For this review, take the finished solid that the model builds, in its own axes (mm). A direction names the side the tool comes from. Round coordinates to 2 decimals unless told otherwise and drop trailing zeros. Write each loop counter-clockwise with the first axis right and the second up, starting at its lowest first coordinate (ties: lowest second). Pieces come first, ordered by that corner, then holes.
from build123d import *

# Parameters (mm, degrees)
ESQUISSE1_R             = 17.7
ESQUISSE1_R_2           = 12.7
BOSS_EXTRU_1_DEPTH      = 12.7
BOSS_EXTRU_2_DEPTH      = 12.7
ESQUISSE3_R             = 3.175
ENL_V_MAT_EXTRU_1_DEPTH = 62.63061651
ESQUISSE4_R             = 3.175
ENL_V_MAT_EXTRU_2_DEPTH = 62.63061651
ESQUISSE5_R             = 3.175
ENL_V_MAT_EXTRU_3_DEPTH = 49.65374434
CONG_1_R                = 1


with BuildPart() as part:
    # Esquisse1 → Boss.-Extru.1 (new body)
    with BuildSketch(Plane.XY):
        Circle(ESQUISSE1_R)
        Circle(ESQUISSE1_R_2, mode=Mode.SUBTRACT)
    extrude(amount=BOSS_EXTRU_1_DEPTH)

    # Esquisse2 → Boss.-Extru.2 (add)
    with BuildSketch(Plane.XY.offset(12.7)):
        Polygon((28.45374434, 23.760125373), (11.133236264, 13.760125373), (6.087254248, 16.620328989), (25.95374434, 28.090252392), align=None)
        Polygon((17.483236264, 2.761602745), (17.437254248, -3.038447676), (37.30374434, 8.431475726), (34.80374434, 12.761602745), align=None)
        Polygon((11.35, -36.521728118), (11.35, -13.581881313), (6.35, -16.521728118), (6.35, -36.521728118), align=None)
        Polygon((-6.35, -16.521728118), (-11.35, -13.581881313), (-11.35, -36.521728118), (-6.35, -36.521728118), align=None)
        Polygon((-37.30374434, 8.431475726), (-17.437254248, -3.038447676), (-17.483236264, 2.761602745), (-34.80374434, 12.761602745), align=None)
        Polygon((-11.133236264, 13.760125373), (-6.087254248, 16.620328989), (-25.95374434, 28.090252392), (-28.45374434, 23.760125373), align=None)
    extrude(amount=-BOSS_EXTRU_2_DEPTH)

    # Esquisse3 → Enlèv. mat.-Extru.1 (cut, through all)
    with BuildSketch(Plane(origin=(5.675, 9.829388333, 0), x_dir=(0.866025404, -0.5, 0), z_dir=(0.5, 0.866025404, 0))):
        with Locations((-28.584228118, -6.35)):
            Circle(ESQUISSE3_R)
    extrude(amount=-ENL_V_MAT_EXTRU_1_DEPTH, mode=Mode.SUBTRACT)

    # Esquisse4 → Enlèv. mat.-Extru.2 (cut, through all)
    with BuildSketch(Plane(origin=(-5.675, 9.829388333, 0), x_dir=(0.866025404, 0.5, 0), z_dir=(-0.5, 0.866025404, 0))):
        with Locations((28.584228118, -6.35)):
            Circle(ESQUISSE4_R)
    extrude(amount=-ENL_V_MAT_EXTRU_2_DEPTH, mode=Mode.SUBTRACT)

    # Esquisse5 → Enlèv. mat.-Extru.3 (cut, through all)
    with BuildSketch(Plane(origin=(11.35, 0, 0), x_dir=(0, 0, -1), z_dir=(1, 0, 0))):
        with Locations((-6.35, -28.584228118)):
            Circle(ESQUISSE5_R)
    extrude(amount=-ENL_V_MAT_EXTRU_3_DEPTH, mode=Mode.SUBTRACT)

    # Congé1
    cong_1_edges = [part.edges().sort_by_distance(p)[0] for p in [
        (25.95374434, 28.090252392, 6.35),
        (28.45374434, 23.760125373, 6.35),
        (11.133236264, 13.760125373, 6.35),
        (6.087254248, 16.620328989, 6.35),
        (17.483236264, 2.761602745, 6.35),
        (34.80374434, 12.761602745, 6.35),
        (37.30374434, 8.431475726, 6.35),
        (17.437254248, -3.038447676, 6.35),
        (11.35, -36.521728118, 6.35),
        (6.35, -36.521728118, 6.35),
        (6.35, -16.521728118, 6.35),
        (11.35, -13.581881313, 6.35),
        (-6.35, -16.521728118, 6.35),
        (-6.35, -36.521728118, 6.35),
        (-11.35, -36.521728118, 6.35),
        (-11.35, -13.581881313, 6.35),
        (-37.30374434, 8.431475726, 6.35),
        (-34.80374434, 12.761602745, 6.35),
        (-17.483236264, 2.761602745, 6.35),
        (-17.437254248, -3.038447676, 6.35),
        (-11.133236264, 13.760125373, 6.35),
        (-28.45374434, 23.760125373, 6.35),
        (-25.95374434, 28.090252392, 6.35),
        (-6.087254248, 16.620328989, 6.35),
    ]]
    fillet(cong_1_edges, radius=CONG_1_R)


solid = part.part
(1) We need section A-A, the plane y = 0. Give the boundary of the cut face in (x, z).
Geometry check:
outline: (-22.7, 0) - (-12.7, 0) - (-12.7, 12.7) - (-22.7, 12.7) - close; (12.7, 0) - (22.7, 0) - (22.7, 12.7) - (12.7, 12.7) - close
(2) We need section C-C, the plane y = -30. Give the boundary of the cut face in (x, z).
Geometry check:
outline: (-11.35, 0) - (-6.35, 0) - (-6.35, 3.51) - (-11.35, 3.51) - close; (-11.35, 9.19) - (-6.35, 9.19) - (-6.35, 12.7) - (-11.35, 12.7) - close; (6.35, 0) - (11.35, 0) - (11.35, 3.51) - (6.35, 3.51) - close; (6.35, 9.19) - (11.35, 9.19) - (11.35, 12.7) - (6.35, 12.7) - close
(3) For pin 1 Ø6.5 at (y, z) = (-22.5, 5) entering from -X; pin 2 Ø5 at (y, z) = (17.5, 4) entering from -X; pin 3 Ø1.5 at (y, z) = (6, 6) entering from -X; pin 4 Ø4 at (y, z) = (-28.58, 6.35) entering from +X, all flat-tipped, find the tip position at first contact; note any pin that passes through.
Geometry check:
pin 1: stops at x = -11.35
pin 2: stops at x = -21.7
pin 3: stops at x = -34.39
pin 4: passes through
(4) We need section B-B, the plane x = 0. Give the boundary of the cut face in (y, z).
Geometry check:
outline: (-17.7, 0) - (-12.7, 0) - (-12.7, 12.7) - (-17.7, 12.7) - close; (12.7, 0) - (17.7, 0) - (17.7, 12.7) - (12.7, 12.7) - close
(5) We need section D-D, the plane z = 7.75. State how many separate pieces and enclosed holes the cut face has, and give its area (3 significant figures).
Geometry check:
separate pieces: 7
enclosed holes: 1
area: 945 mm2
(6) For faces 4 (the face through (15.656, 22.145, 6.439)), 5 (the face through (11.35, -25, 6)), 6 (the face through (15.364, 8.788, 6.261)), list the 3-axis set-ups (+Z, -Z, +X, -X, +Y, -Y) from which the entire face can be reached by the end or side of a thin tool; tool diameter is ignored.
Geometry check:
face 4: +Z, -Z, +Y
face 5: +Z, -Z, +X, -Y
face 6: +Z, -Z
(7) Mouldability with a two-part tool opening along Z and no side actions: class faces 1 (the face through (0.1, 17.7, 6.3)), 2 (the face through (11, -7, 12.7)), 3 (the face through (-31.91, 8.24, 6.21)) as pulls with the +Z half, pulls with the -Z half, needs draft (parallel to the pull), parting line crosses it, or undercut.
Geometry check:
face 1: needs draft
face 2: pulls with the +Z half
face 3: undercut
(8) For line 1 along Y through (x, z) = (7.55, 6.35); line 2 along Y through (x, z) = (-8.75, 6.35); line 3 along X through (y, z) = (11, 1.5), list the stretches that pass through material, from the lowest coordinate up.
Geometry check:
line 1: y = -36.52 to -31.76, -25.41 to -10.21, 10.21 to 17.46
line 2: y = -36.52 to -31.76, -25.41 to -9.2, 9.2 to 18.16
line 3: x = -35.82 to -31.75, -13.87 to -6.35, 6.35 to 13.87, 31.75 to 35.82
